Autodesk Inventor part; units mm, degrees
ref_plane "YZ Plane" through (0, 0, 0) normal (1, 0, 0) x (0, 1, 0)
ref_plane "XZ Plane" through (0, 0, 0) normal (0, 1, 0) x (-1, 0, 0)
ref_plane "XY Plane" through (0, 0, 0) normal (0, 0, 1) x (1, 0, 0)
sketch "스케치1" plane through (0, 0, 0) normal (0, 0, 1) x (1, 0, 0)
  circle A0 centre (-80.3814, -83.6055) radius 3
  circle A1 centre (-80.3814, -83.6055) radius 1.5
  circle A2 centre (-95.5814, -68.4055) radius 3
  circle A3 centre (-95.5814, -68.4055) radius 1.5
  line L0 (-78.3814, -66.4055) -> (-97.5814, -66.4055)
  line L1 (-97.5814, -66.4055) -> (-97.5814, -85.6055)
  line L2 (-97.5814, -85.6055) -> (-78.3814, -85.6055)
  line L3 (-78.3814, -85.6055) -> (-78.3814, -66.4055)
  point P0 (0, 0)
  dimension "d0" = 19.2
  dimension "d1" = 19.2
  dimension "d2" = 2
  dimension "d3" = 2
extrude "돌출1" add sketch "스케치1" along normal blind 1.6 contours L3 L2 A0 | A0 L2 L1 A2 L0 L3 | A2 L1 L0 picked at (-80.5204, -85.4352) picked at (-95.563, -66.5758)
sketch "스케치2" plane through (0, 0, 1.6) normal (0, 0, 1) x (1, 0, 0)
  line L0 (-78.9814, -67.0055) -> (-96.9814, -67.0055)
  line L1 (-96.9814, -67.0055) -> (-96.9814, -85.0055)
  line L2 (-96.9814, -85.0055) -> (-78.9814, -85.0055)
  line L3 (-78.9814, -85.0055) -> (-78.9814, -67.0055)
  line L4 (-97.5814, -85.6055) -> (-78.3814, -85.6055)
  line L5 (-78.3814, -85.6055) -> (-78.3814, -66.4055)
  line L6 (-78.3814, -66.4055) -> (-97.5814, -66.4055)
  line L7 (-97.5814, -66.4055) -> (-97.5814, -85.6055)
  circle A0 centre (-80.3814, -83.6055) radius 1.5
  circle A1 centre (-95.5814, -68.4055) radius 1.5
  point P0 (0, 0)
  dimension "d6" = 18
  dimension "d7" = 18
  dimension "d8" = 19.2
  dimension "d9" = 0.6
  dimension "d10" = 0.6
extrude "돌출2" add sketch "스케치2" along normal blind 5 contours L3 A0 L2 L1 A1 L0 | A1 L1 L0 | L3 A0 L2 | A1 L1 L0 | L3 L2 A0
sketch "스케치3" plane through (0, 0, 6.6) normal (0, 0, 1) x (1, 0, 0)
  line L0 (-96.9814, -85.0055) -> (-78.9814, -85.0055)
  line L1 (-78.9814, -85.0055) -> (-78.9814, -67.0055)
  line L2 (-78.9814, -67.0055) -> (-96.9814, -67.0055)
  line L3 (-96.9814, -67.0055) -> (-96.9814, -85.0055)
  point P0 (0, 0)
extrude "돌출3" add sketch "스케치3" along normal blind 10 draft -10
properties part number "KeySwitch"
Input: part model. Units: mm. Frame: model coordinates. A direction names the side the tool comes from. Round coordinates to 2 decimals unless told otherwise and drop trailing zeros. Loops run counter-clockwise (first coordinate to the right, second up) from the corner with the lowest first, then second, coordinate; pieces in that order, holes last.
1) Section query A-A on x = -87.5. Return the cut outline in (y, z), plus the area to 3 significant figures.
Ans:
outline: (-85.61, 0) - (-66.41, 0) - (-66.41, 1.6) - (-67.01, 1.6) - (-67.01, 6.6) - (-68.77, 16.6) - (-83.24, 16.6) - (-85.01, 6.6) - (-85.01, 1.6) - (-85.61, 1.6) - close
area: 283 mm2
2) Section query B-B on y = -76.25. Return the cut outline in (x, z).
Ans:
outline: (-97.58, 0) - (-78.38, 0) - (-78.38, 1.6) - (-78.98, 1.6) - (-78.98, 6.6) - (-80.74, 16.6) - (-95.22, 16.6) - (-96.98, 6.6) - (-96.98, 1.6) - (-97.58, 1.6) - close
3) Material intervals for line 1 (Y direction, x = -91.75, z = 2.5); line 2 (Y direction, x = -81.5, z = 1); line 3 (X direction, y = -68, z = 6), sorted ascending.
Ans:
line 1: y = -85.01 to -67.01
line 2: y = -85.61 to -84.6, -82.61 to -66.41
line 3: x = -96.98 to -78.98
4) Section query C-C on z = 8.75. Return the cut outline in (x, y), plus the area to 3 significant figures.
Ans:
outline: (-96.6, -84.63) - (-79.36, -84.63) - (-79.36, -67.38) - (-96.6, -67.38) - close
area: 297 mm2
5) Set-up query: faces 1 (the flat face through (-78.981, -76, 4)), 2 (the flat face through (-88, -85.006, 4)), 3 (the flat face through (-88, -76, 16.6)), 4 (the flat face through (-96.981, -76, 4)), 5 (the flat face through (-96, -68, 1.6)). Return all of +Z, -Z, +X, -X, +Y, -Y with unobstructed straight access to the full face (end or side cutting, diameter ignored); none if empty.
Ans:
face 1: +Z, +X, +Y, -Y
face 2: +Z, +X, -X, -Y
face 3: +Z, +X, -X, +Y, -Y
face 4: +Z, -X, +Y, -Y
face 5: -Z
6) Section query D-D on y = -82.75. Return the cut outline in (x, z).
Ans:
outline: (-97.58, 0) - (-81.61, 0) - (-81.61, 1.6) - (-79.15, 1.6) - (-79.15, 0) - (-78.38, 0) - (-78.38, 1.6) - (-78.98, 1.6) - (-78.98, 6.6) - (-80.74, 16.6) - (-95.22, 16.6) - (-96.98, 6.6) - (-96.98, 1.6) - (-97.58, 1.6) - close
7) Pin query (flat end, axial travel): pin 1 (1 mm diameter, centred on x = -80.5, z = 14, fed in from -Y); pin 2 (2.5 mm diameter, centred on x = -91.5, z = 4, fed in from -Y); pin 3 (1.5 mm diameter, centred on x = -80, y = -83, fed in from -Z). Return the tip coordinate at first contact, or that it passes through.
Ans:
pin 1: stops at y = -83.79
pin 2: stops at y = -85.01
pin 3: stops at z = 1.6
8) Pull-direction query (Y, two-part tool) for faces 6 (the flat face through (-80, -84, 1.6)), 7 (the flat face through (-88, -67.006, 4)), 8 (the flat face through (-79.85, -75.88, 11.53)); classes: released by +Y, released by -Y, zero draft, split by the parting line, or undercut.
Ans:
face 6: undercut
face 7: released by +Y
face 8: zero draft
